from build123d import *

# Parameters (mm, degrees)
F0_R     = 3.302
F0_R_2   = 1.7
F0_R_3   = 18
F1_DEPTH = 12.7
F2_DEPTH = 25.4
F3_R     = 6.35
F4_R     = 2.7051
F5_DEPTH = 25.4


# Not quite as in the source:
# - a feature names something its author has since deleted; it is built from what else it names


with BuildPart() as f1:
    # F0 (on Front) → F1 (new body)
    with BuildSketch(Plane.XZ):
        with BuildLine():
            Line((108.4265169831, 0.0004552842), (32.2265169831, 152.4004552842))
            Line((32.2265169831, 152.4004552842), (-107.4734830169, 152.4004552842))
            Line((-107.4734830169, 152.4004552842), (-107.4734830169, -76.1995447158))
            add(Edge.make_bspline(
                [(-82.0734830169, -114.2995447158), (-82.8863746009, -95.7832909802), (-85.4194185281, -76.1871889735), (-107.4734830169, -76.1995447158)],
                knots=[0, 0, 0, 0, 45.7905011984, 45.7905011984, 45.7905011984, 45.7905011984], degree=3))
            Line((-82.0734830169, -114.2995447158), (108.4265169831, -114.2995447158))
            Line((108.4265169831, -114.2995447158), (108.4265169831, 0.0004552842))
        make_face()
        with Locations((-88.4234830169, -57.1371889735)):
            Circle(F0_R, mode=Mode.SUBTRACT)
        with Locations((-88.4234830169, -19.0371889735)):
            Circle(F0_R, mode=Mode.SUBTRACT)
        with Locations((-92.9944827628, 14.5430932346)):
            Circle(F0_R_2, mode=Mode.SUBTRACT)
        with Locations((-69.4244827628, 16.1130932346)):
            Circle(F0_R_2, mode=Mode.SUBTRACT)
        with Locations((-45.8544827628, 14.5430932346)):
            Circle(F0_R_2, mode=Mode.SUBTRACT)
        with Locations((-91.4244827628, 38.1130932346)):
            Circle(F0_R_2, mode=Mode.SUBTRACT)
        with Locations((-69.4244827628, 38.1130932346)):
            Circle(F0_R_3, mode=Mode.SUBTRACT)
        with Locations((-92.9944827628, 61.6830932346)):
            Circle(F0_R_2, mode=Mode.SUBTRACT)
        with Locations((-69.4244827628, 60.1130932346)):
            Circle(F0_R_2, mode=Mode.SUBTRACT)
        with Locations((-47.4244827628, 38.1130932346)):
            Circle(F0_R_2, mode=Mode.SUBTRACT)
        with Locations((-45.8544827628, 61.6830932346)):
            Circle(F0_R_2, mode=Mode.SUBTRACT)
        with Locations((-88.4234830169, 95.2504552842)):
            Circle(F0_R, mode=Mode.SUBTRACT)
        with Locations((-88.4234830169, 133.3504552842)):
            Circle(F0_R, mode=Mode.SUBTRACT)
    extrude(amount=F1_DEPTH)

    # F0 (on Front) → F2 (cut)
    with BuildSketch(Plane.XZ):
        with BuildLine():
            add(Edge.make_bspline(
                [(-82.0734830169, -114.2995447158), (-82.8863746009, -95.7832909802), (-85.4194185281, -76.1871889735), (-107.4734830169, -76.1995447158)],
                knots=[0, 0, 0, 0, 45.7905011984, 45.7905011984, 45.7905011984, 45.7905011984], degree=3))
            Line((-107.4734830169, -76.1995447158), (-107.4734830169, -114.2995447158))
            Line((-107.4734830169, -114.2995447158), (-82.0734830169, -114.2995447158))
        make_face()
        with BuildLine():
            Line((108.4265169831, 0.0004552842), (32.2265169831, 152.4004552842))
            Line((32.2265169831, 152.4004552842), (-107.4734830169, 152.4004552842))
            Line((-107.4734830169, 152.4004552842), (-107.4734830169, -76.1995447158))
            add(Edge.make_bspline(
                [(-82.0734830169, -114.2995447158), (-82.8863746009, -95.7832909802), (-85.4194185281, -76.1871889735), (-107.4734830169, -76.1995447158)],
                knots=[0, 0, 0, 0, 45.7905011984, 45.7905011984, 45.7905011984, 45.7905011984], degree=3))
            Line((-82.0734830169, -114.2995447158), (108.4265169831, -114.2995447158))
            Line((108.4265169831, -114.2995447158), (108.4265169831, 0.0004552842))
        make_face()
        with Locations((-88.4234830169, -57.1371889735)):
            Circle(F0_R, mode=Mode.SUBTRACT)
        with Locations((-88.4234830169, -19.0371889735)):
            Circle(F0_R, mode=Mode.SUBTRACT)
        with Locations((-92.9944827628, 14.5430932346)):
            Circle(F0_R_2, mode=Mode.SUBTRACT)
        with Locations((-69.4244827628, 16.1130932346)):
            Circle(F0_R_2, mode=Mode.SUBTRACT)
        with Locations((-45.8544827628, 14.5430932346)):
            Circle(F0_R_2, mode=Mode.SUBTRACT)
        with Locations((-91.4244827628, 38.1130932346)):
            Circle(F0_R_2, mode=Mode.SUBTRACT)
        with Locations((-69.4244827628, 38.1130932346)):
            Circle(F0_R_3, mode=Mode.SUBTRACT)
        with Locations((-92.9944827628, 61.6830932346)):
            Circle(F0_R_2, mode=Mode.SUBTRACT)
        with Locations((-69.4244827628, 60.1130932346)):
            Circle(F0_R_2, mode=Mode.SUBTRACT)
        with Locations((-47.4244827628, 38.1130932346)):
            Circle(F0_R_2, mode=Mode.SUBTRACT)
        with Locations((-45.8544827628, 61.6830932346)):
            Circle(F0_R_2, mode=Mode.SUBTRACT)
        with Locations((-88.4234830169, 95.2504552842)):
            Circle(F0_R, mode=Mode.SUBTRACT)
        with Locations((-88.4234830169, 133.3504552842)):
            Circle(F0_R, mode=Mode.SUBTRACT)
    extrude(amount=-F2_DEPTH, mode=Mode.SUBTRACT)

    # F3
    f3_edges = [f1.edges().sort_by_distance(p)[0] for p in [
        (-107.473483, -6.35, -76.199545),
        (-107.473483, -6.35, 152.400455),
        (108.426517, -6.35, 0.000455),
        (32.226517, -6.35, 152.400455),
    ]]
    fillet(f3_edges, radius=F3_R)

    # F4 (on face) → F5 (cut)
    with BuildSketch(Plane(origin=(0, 0, -114.2995447158), x_dir=(1, 0, 0), z_dir=(0, 0, -1))):
        with Locations((-70.4482253863, 6.35)):
            Circle(F4_R)
        with Locations((-29.1732253863, 6.35)):
            Circle(F4_R)
        with Locations((12.1017746137, 6.35)):
            Circle(F4_R)
        with Locations((53.3767746137, 6.35)):
            Circle(F4_R)
        with Locations((94.6517746137, 6.35)):
            Circle(F4_R)
    extrude(amount=-F5_DEPTH, mode=Mode.SUBTRACT)


solid = f1.part
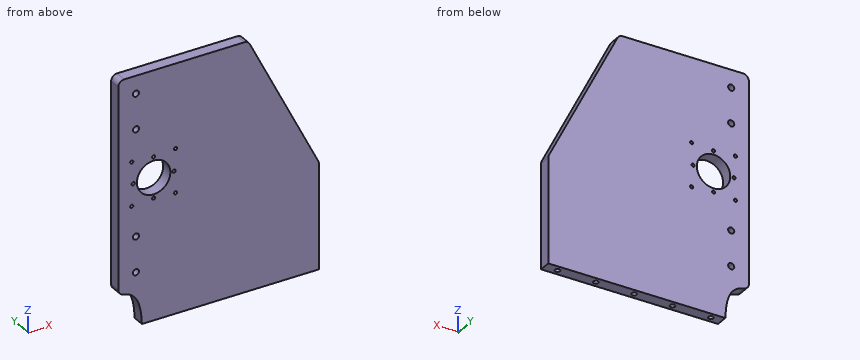
CAD build for the part. Positions are in the model's coordinates, mm. Round coordinates to 2 decimals unless told otherwise and drop trailing zeros. Loops run counter-clockwise (first coordinate to the right, second up) from the corner with the lowest first, then second, coordinate; pieces in that order, holes last.
(1) Cut at C-C (y = -6.35). State how many separate pieces and enclosed holes the cut face has, plus the area to 3 significant figures.
(2) Cut at B-B (x = 62.5). Give the cut face in (y, z), plus the area to 3 significant figures.
(3) Cut at A-A (z = 23). Give the cut face in (x, y), plus the area to 3 significant figures.
(4) Wall check: line 1 along Z through (x, y) = (-68, -1); line 2 along X through (y, z) = (-6.35, -94.25); line 3 along Z through (x, y) = (-64.5, -1.5). Give the ranges that are in metal, low to high.
(5) Drop flat-ended pins along their axis: pin 1 (4.5 mm diameter, centred on x = 53.38, y = -6.35, fed in from +Z); pin 2 (1.6 mm diameter, centred on x = -30, y = -6.5, fed in from -Z); pin 3 (6 mm diameter, centred on x = 94.65, y = -6.35, fed in from +Z). Give the stop position or say it passes through.
Findings below:
1. separate pieces: 1
1. enclosed holes: 13
1. area: 49,000 mm2
2. outline: (-12.7, -114.3) - (0, -114.3) - (0, 91.85) - (-12.7, 91.85) - close
2. area: 2,620 mm2
3. outline: (-107.47, -12.7) - (-79.2, -12.7) - (-79.2, 0) - (-107.47, 0) - close; (-59.65, -12.7) - (96.93, -12.7) - (96.93, 0) - (-59.65, 0) - close
3. area: 2,350 mm2
4. line 1: z = -114.3 to 15.19, 17.04 to 20.17, 56.06 to 59.19, 61.04 to 152.4
4. line 2: x = -84.61 to -73.15, -67.74 to -31.88, -26.47 to 9.4, 14.81 to 50.67, 56.08 to 91.95, 97.36 to 108.43
4. line 3: z = -114.3 to 20.8, 55.43 to 152.4
5. pin 1: stops at z = 114.59
5. pin 2: stops at z = -88.9
5. pin 3: stops at z = 33.55
